Job drawing, mm, ordinate dimensions from the low corner. One solid piece. A direction names the side the tool comes from. Round coordinates to 2 decimals unless told otherwise and drop trailing zeros. Write each loop counter-clockwise with the first axis right and the second up, starting at its lowest first coordinate (ties: lowest second). Pieces come first, ordered by that corner, then holes. Notation, with made-up numbers: (-29, 14) - (-21, 14) arc R28 ccw to (-21, 38) - close; hole circle Ø7 at (77.5, -20). An arc over 180 degrees is marked (long way). Write each question's results on one line, items separated by ' | '.
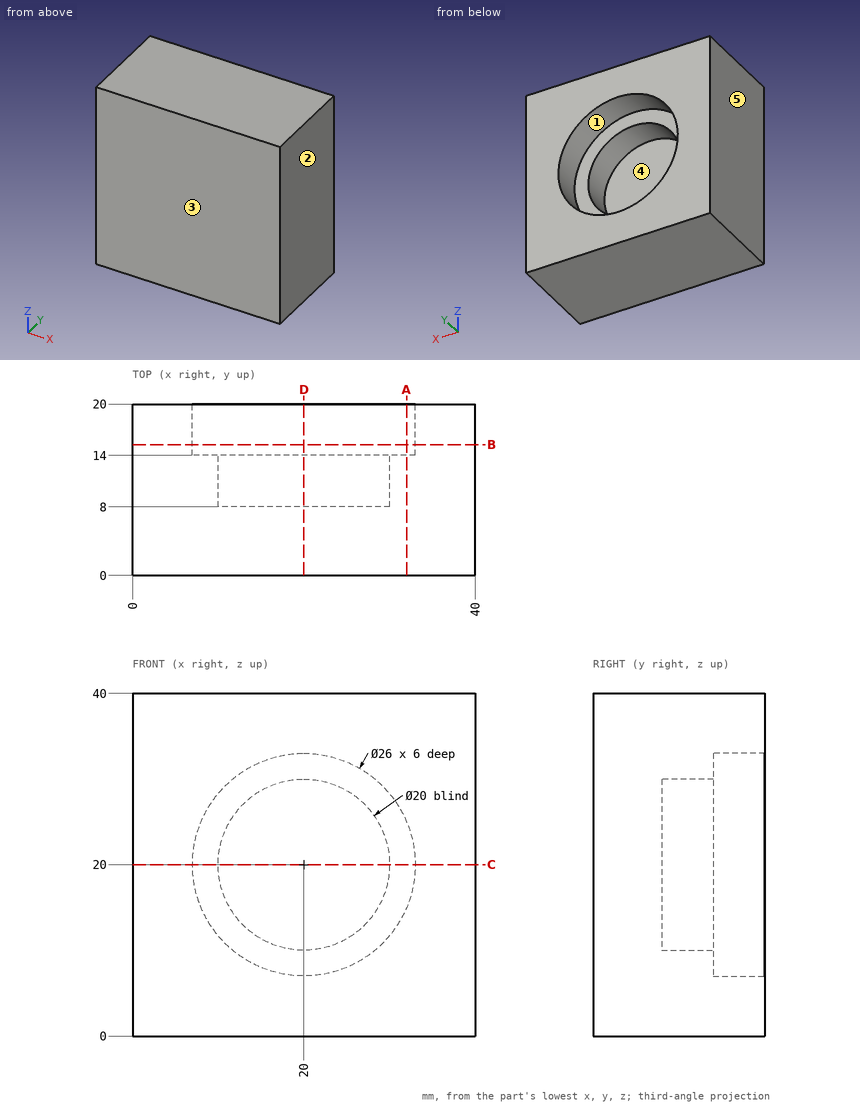
(1) Two-plate mould, pull along X, no slides. Class the marked faces 3, 4 and 5: released by +X, released by -X, zero draft, split by the parting line, or undercut.
Worked answers:
face 3: zero draft | face 4: undercut | face 5: released by -X
(2) Tool access for the marked faces 1 and 2: list every direction of +Z, -Z, +X, -X, +Y, -Y with a clear straight run to the whole face (end or side of a thin tool).
Worked answers:
face 1: +Y | face 2: +Z, -Z, +X, +Y, -Y
(3) Slice it at D-D, the plane x = 20. Write the cut outline in (y, z).
Worked answers:
outline: (0, 0) - (20, 0) - (20, 7) - (14, 7) - (14, 10) - (8, 10) - (8, 30) - (14, 30) - (14, 33) - (20, 33) - (20, 40) - (0, 40) - close
(4) Flat gauge pins, fed straight in: pin 1 Ø6 at (x, z) = (13, 15.5) entering from +Y; pin 2 Ø13 at (x, z) = (18.5, 19) entering from +Y. Where does each tip first touch, or does it go through?
Worked answers:
pin 1: stops at y = 14 | pin 2: stops at y = 8
(5) Slice it at A-A, the plane x = 32. Write the cut outline in (y, z), and give its area (3 significant figures).
Worked answers:
outline: (0, 0) - (20, 0) - (20, 15) - (14, 15) - (14, 25) - (20, 25) - (20, 40) - (0, 40) - close | area: 740 mm2
(6) Drill centre lines: probe 1 along X at (y, z) = (10.1, 20); probe 2 along X at (y, z) = (17.55, 20); probe 3 along Y at (x, z) = (20.5, 25). Where is each one in solid material? Low to high. Write a range as [from, to].
Worked answers:
probe 1: x = [0, 10], [30, 40] | probe 2: x = [0, 7], [33, 40] | probe 3: y = [0, 8]
(7) Slice it at B-B, the plane y = 15.25. Write the cut outline in (x, z).
Worked answers:
outline: (0, 0) - (40, 0) - (40, 40) - (0, 40) - close; hole circle Ø26 at (20, 20)
(8) Slice it at C-C, the plane z = 20. Write the cut outline in (x, y).
Worked answers:
outline: (0, 0) - (40, 0) - (40, 20) - (33, 20) - (33, 14) - (30, 14) - (30, 8) - (10, 8) - (10, 14) - (7, 14) - (7, 20) - (0, 20) - close
